Autodesk Inventor part; units mm, degrees
ref_plane "YZ Plane" through (0, 0, 0) normal (1, 0, 0) x (0, 1, 0)
ref_plane "XZ Plane" through (0, 0, 0) normal (0, 1, 0) x (-1, 0, 0)
ref_plane "XY Plane" through (0, 0, 0) normal (0, 0, 1) x (1, 0, 0)
sketch "Sketch1" plane through (0, 0, 0) normal (0, 1, 0) x (-1, 0, 0)
  circle A0 centre (0, 0) radius 15
  dimension "d0" = 30
extrude "Extrusion1" add sketch "Sketch1" along normal blind 60
sketch "Sketch2" plane through (0, 60, 0) normal (0, 1, 0) x (1, 0, 0)
  arc A0 (-3.8268, -9.2388) -> (0, -10) centre (0, 0) ccw
  line L0 (0, -10) -> (0, -15)
  circle A1 centre (0, 0) radius 15
  line L1 (-3.8268, -9.2388) -> (-5.7403, -13.8582)
  arc A2 (-5.7403, -13.8582) -> (0, -15) centre (0, 0) ccw
  arc A3 (3.8268, -9.2388) -> (7.0711, -7.0711) centre (0, 0) ccw
  line L2 (7.0711, -7.0711) -> (10.6066, -10.6066)
  line L3 (3.8268, -9.2388) -> (5.7403, -13.8582)
  arc A4 (5.7403, -13.8582) -> (10.6066, -10.6066) centre (0, 0) ccw
  arc A5 (9.2388, -3.8268) -> (10, 0) centre (0, 0) ccw
  line L4 (10, 0) -> (15, 0)
  line L5 (9.2388, -3.8268) -> (13.8582, -5.7403)
  arc A6 (13.8582, -5.7403) -> (15, 0) centre (0, 0) ccw
  arc A7 (9.2388, 3.8268) -> (7.0711, 7.0711) centre (0, 0) ccw
  line L6 (7.0711, 7.0711) -> (10.6066, 10.6066)
  line L7 (9.2388, 3.8268) -> (13.8582, 5.7403)
  arc A8 (13.8582, 5.7403) -> (10.6066, 10.6066) centre (0, 0) ccw
  arc A9 (3.8268, 9.2388) -> (0, 10) centre (0, 0) ccw
  line L8 (0, 10) -> (0, 15)
  line L9 (3.8268, 9.2388) -> (5.7403, 13.8582)
  arc A10 (5.7403, 13.8582) -> (0, 15) centre (0, 0) ccw
  arc A11 (-3.8268, 9.2388) -> (-7.0711, 7.0711) centre (0, 0) ccw
  line L10 (-7.0711, 7.0711) -> (-10.6066, 10.6066)
  line L11 (-3.8268, 9.2388) -> (-5.7403, 13.8582)
  arc A12 (-5.7403, 13.8582) -> (-10.6066, 10.6066) centre (0, 0) ccw
  arc A13 (-9.2388, 3.8268) -> (-10, 0) centre (0, 0) ccw
  line L12 (-10, 0) -> (-15, 0)
  line L13 (-9.2388, 3.8268) -> (-13.8582, 5.7403)
  arc A14 (-13.8582, 5.7403) -> (-15, 0) centre (0, 0) ccw
  arc A15 (-9.2388, -3.8268) -> (-7.0711, -7.0711) centre (0, 0) ccw
  line L14 (-7.0711, -7.0711) -> (-10.6066, -10.6066)
  line L15 (-9.2388, -3.8268) -> (-13.8582, -5.7403)
  arc A16 (-13.8582, -5.7403) -> (-10.6066, -10.6066) centre (0, 0) ccw
  point P0 (15, 0)
  dimension "d3" = 20
  dimension "d7" = 360
extrude "Extrusion2" cut sketch "Sketch2" against normal blind 5 contours L1 A1 L14 A15 L15 L12 A13 L13 L10 A11 L11 L8 A9 L9 L6 A7 L7 L4 A5 L5 L2 A3 L3 L0 A0
sketch "Sketch3" plane through (0, 0, 0) normal (1, 0, 0) x (0, 1, 0)
  line L0 (0, 15) -> (60, 15)
  line L1 (55, -13.8582) -> (55, -15)
  line L2 (0, -15) -> (60, -15)
  line L3 (50, -15) -> (46.4645, -11.4645)
  line L4 (0, -15) -> (0, 15)
  line L5 (0, -15) -> (5, -15)
  line L6 (5, -15) -> (8.5355, -11.4645)
  line L7 (8.5355, -11.4645) -> (46.4645, -11.4645)
  line L8 (46.4645, -11.4645) -> (8.5355, -11.4645)
  line L9 (50, -15) -> (50, -20)
  line L10 (50, -20) -> (5, -20)
  line L11 (5, -20) -> (5, -15)
  line L12 (0, 0) -> (62.9673, 0)
  dimension "d13" = 5
  dimension "d16" = 5
  dimension "d17" = 5
revolve "Revolution1" cut sketch "Sketch3" angle 360 about axis through (0, 0, 0) along (0, 1, 0)
sketch "Sketch4" plane through (0, 0, 0) normal (0, -1, 0) x (1, 0, 0)
  circle A0 centre (0, 0) radius 11.4645
  circle A1 centre (0, 0) radius 2.5
  dimension "d19" = 5
extrude "Extrusion3" cut sketch "Sketch4" against normal blind 4 contours A1
sketch "Sketch5" plane through (0, 55, 0) normal (0, 1, 0) x (1, 0, 0)
  line L0 (-2.5, 2.5) -> (2.5, 2.5)
  line L1 (2.5, 2.5) -> (2.5, -2.5)
  line L2 (2.5, -2.5) -> (-2.5, -2.5)
  line L3 (-2.5, -2.5) -> (-2.5, 2.5)
  point P0 (0, 0)
  dimension "d22" = 2.5
  dimension "d23" = 2.5
  dimension "d24" = 2.5
  dimension "d25" = 2.5
extrude "Extrusion4" cut sketch "Sketch5" against normal blind 7
properties part number "TowerUntagged"
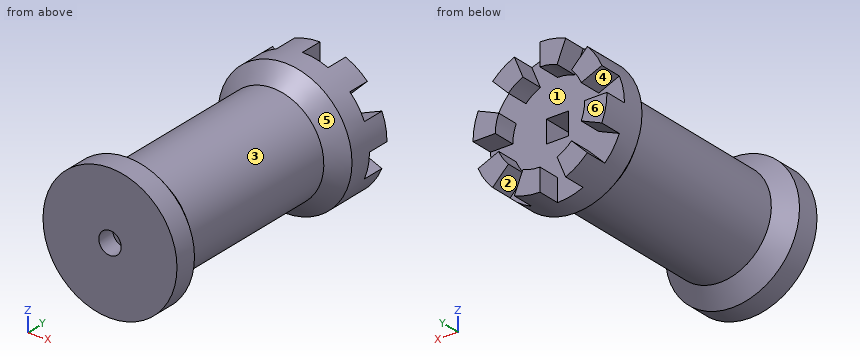
Input: part model. Units: mm. Frame: model coordinates. Face numbers are marked on the shaded views. A direction names the side the tool comes from. Coordinates: 2 decimals unless noted, no trailing zeros. Loops run counter-clockwise (first coordinate to the right, second up) from the corner with the lowest first, then second, coordinate; pieces in that order, holes last.
(1) Section A-A on y = 34.5. Return the cut outline in (x, z), then the cut area to 3 significant figures.
(2) Set-up query: the marked faces 1, 2 and 3. Return all of +Z, -Z, +X, -X, +Y, -Y with unobstructed straight access to the full face (end or side cutting, diameter ignored); none if empty.
(3) Pull-direction query (Y, two-part tool) for the marked faces 4, 5 and 6; classes: released by +Y, released by -Y, zero draft, split by the parting line, or undercut.
(4) First-contact query: pin 1 Ø5 at (x, y) = (-1.5, 24.5) entering from -Z; pin 2 Ø5 at (x, y) = (-8.5, 14.5) entering from -Z; pin 3 Ø2.5 at (y, z) = (58, 13.5) entering from +X. Flat tips, straight axial feed; report the tip coordinate or a pass-through.
(5) Material intervals for probe 1 along Z at (x, y) = (0, 1.8); probe 2 along Y at (x, z) = (-5.75, 9.25); probe 3 along Z at (x, y) = (0.5, 34.5), sorted ascending.
Data:
1. outline: circle Ø22.93 at (0, 0)
1. area: 413 mm2
2. face 1: +Y
2. face 2: -Z, +Y
2. face 3: none
3. face 4: zero draft
3. face 5: undercut
3. face 6: released by +Y
4. pin 1: stops at z = -11.46
4. pin 2: stops at z = -9.77
4. pin 3: stops at x = 8.66
5. probe 1: z = -15 to -2.5, 2.5 to 15
5. probe 2: y = 0 to 55
5. probe 3: z = -11.45 to 11.45
